Source: CAD feature listing. Evaluate the final solid. Frame: model axes, mm. Face numbers are marked on the shaded views. A direction names the side the tool comes from. Coordinates: 2 decimals unless noted, no trailing zeros. Loops run counter-clockwise (first coordinate to the right, second up) from the corner with the lowest first, then second, coordinate; pieces in that order, holes last.
Item 1: Reachability of the marked faces 1, 2 and 3 from +Z, -Z, +X, -X, +Y, -Y: full face, straight path, thin tool, end or side. Return the list, or none.
Item 2: Line query: probe 1 along Y at (x, z) = (-6, -8.5); probe 2 along X at (y, z) = (227.5, -0.5); probe 3 along Y at (x, z) = (3, 9). Output: solid intervals per line, ascending.
Item 3: Section query A-A, the plane z = 0. Return the cut outline in (x, y), then the cut area to 3 significant figures.
Item 4: Section query B-B, the plane y = 203.5. Return the cut outline in (x, z), then the cut area to 3 significant figures.
Item 5: Pin query (flat end, axial travel): pin 1 Ø1 at (x, y) = (2, 102) entering from -Z; pin 2 Ø4 at (x, y) = (0, 224) entering from +Z; pin 3 Ø10 at (x, y) = (-6, 221.5) entering from +Z; pin 4 Ø12.5 at (x, z) = (0.5, 5.5) entering from +Y. Return the tip coordinate at first contact, or that it passes through.
```python
from build123d import *

# Parameters (mm, degrees)
SKETCH_1_R          = 12.5
EXTRUDE_1_DEPTH     = 196.5
SKETCH_2_R          = 10
EXTRUDE_2_DEPTH     = 15
EXTRUDE_START       = 45
SKETCH_3_R          = 10
EXTRUDE_3_DEPTH     = 45
SKETCH_4_R          = 6
EXTRUDE_4_DEPTH     = 23
CUT_EXTRUDE_1_DEPTH = 4
CHAMFER_1_SIZE      = 1
SKETCH_6_W          = 0.5
SKETCH_6_H          = 1


with BuildPart() as part:
    # 草图1 → 凸台-拉伸1 (new body)
    with BuildSketch(Plane(origin=(0, 0, 0), x_dir=(1, 0, 0), z_dir=(0, 1, 0))):
        with Locations(Location((0, 0, 0), (0, 0, 270))):
            Circle(SKETCH_1_R)
    extrude(amount=EXTRUDE_1_DEPTH)

    # 草图2 → 凸台-拉伸2 (add)
    with BuildSketch(Plane.XZ):
        with Locations(Location((0, 0, 0), (0, 0, 270))):
            Circle(SKETCH_2_R)
    extrude(amount=EXTRUDE_2_DEPTH)

    # 草图3 → 凸台-拉伸3 (add)
    with BuildSketch(Plane(origin=(0, 196.5, 0), x_dir=(1, 0, 0), z_dir=(0, 1, 0)).offset(EXTRUDE_START)):
        with Locations(Location((0, 0, 0), (0, 0, 90))):
            Circle(SKETCH_3_R)
    extrude(amount=-EXTRUDE_3_DEPTH)

    # 草图4 → 凸台-拉伸4 (add)
    with BuildSketch(Plane(origin=(0, 241.5, 0), x_dir=(1, 0, 0), z_dir=(0, 1, 0))):
        with Locations(Location((0, 0, 0), (0, 0, 270))):
            Circle(SKETCH_4_R)
    extrude(amount=EXTRUDE_4_DEPTH)

    # 草图5 → 切除-拉伸1 (cut)
    with BuildSketch(Plane(origin=(0, 0, 9.5), x_dir=(-1, 0, 0), z_dir=(0, 0, -1))):
        with BuildLine():
            Line((2, 256.5), (2, 248.5))
            ThreePointArc((2, 248.5), (0, 246.5), (-2, 248.5))
            Line((-2, 248.5), (-2, 256.5))
            ThreePointArc((-2, 256.5), (0, 258.5), (2, 256.5))
        make_face()
    extrude(amount=CUT_EXTRUDE_1_DEPTH, mode=Mode.SUBTRACT)

    # 倒角1
    chamfer_1_edges = [part.edges().sort_by_distance(p)[0] for p in [
        (0, 264.5, -6),
    ]]
    chamfer(chamfer_1_edges, length=CHAMFER_1_SIZE)

    # 草图6 → 切除-旋转1 (revolve, cut)
    with BuildSketch(Plane(origin=(0, 0, 0), x_dir=(0, 0, -1), z_dir=(1, 0, 0))):
        with Locations((5.75, 261)):
            Rectangle(SKETCH_6_W, SKETCH_6_H)
    revolve(axis=Axis((0, 264.5, 0), (0, 1, 0)), mode=Mode.SUBTRACT)


solid = part.part
```
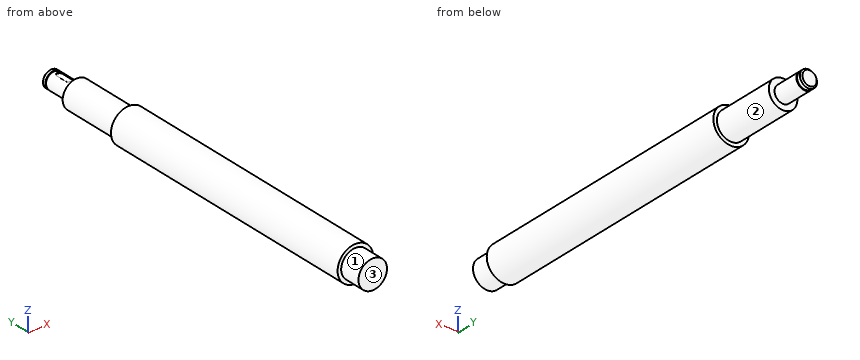
Verdict:
1. face 1: -Y
1. face 2: +Y
1. face 3: +Z, -Z, +X, -X, -Y
2. probe 1: y = 0 to 196.5
2. probe 2: x = -9.99 to 9.99
2. probe 3: y = -15 to 241.5
3. outline: (-12.5, 0) - (-10, 0) - (-10, -15) - (10, -15) - (10, 0) - (12.5, 0) - (12.5, 196.5) - (10, 196.5) - (10, 241.5) - (6, 241.5) - (6, 260.5) - (5.5, 260.5) - (5.5, 261.5) - (6, 261.5) - (6, 263.5) - (5, 264.5) - (-5, 264.5) - (-6, 263.5) - (-6, 261.5) - (-5.5, 261.5) - (-5.5, 260.5) - (-6, 260.5) - (-6, 241.5) - (-10, 241.5) - (-10, 196.5) - (-12.5, 196.5) - close
3. area: 6,390 mm2
4. outline: circle Ø20 at (0, 0)
4. area: 314 mm2
5. pin 1: stops at z = -12.41
5. pin 2: stops at z = 10
5. pin 3: stops at z = 9.95
5. pin 4: stops at y = 264.5
